Work out the finished part from the listing and answer in its coordinate system (mm). Face numbers are marked on the shaded views. A direction names the side the tool comes from. Give positions to 0.01 mm unless a question says otherwise; leave off trailing zeros. Loops run counter-clockwise (first coordinate to the right, second up) from the corner with the lowest first, then second, coordinate; pieces in that order, holes last. Notation, with made-up numbers: M 61.25,5 L 112.25,5 A12 ccw 112.25,11 Z; hole C 82.5,-7 d2. An arc over 180 degrees is marked long. Use a Markdown table: item, result.
```python
from build123d import *

# Parameters (mm, degrees)
F0_W      = 12
F0_H      = 64
F1_DEPTH  = 2
F2_W      = 2
F2_H      = 32
F3_DEPTH  = 8
F4_W      = 2
F4_H      = 32
F5_DEPTH  = 8
F6_W      = 5
F6_H      = 2
F7_DEPTH  = 5
F8_W      = 5
F8_H      = 1
F9_DEPTH  = 16.501
F10_W     = 2
F10_H     = 32
F11_DEPTH = 24
F12_R     = 1.5
F13_DEPTH = 28.001


with BuildPart() as f1:
    # F0 (on Front) → F1 (new body)
    with BuildSketch(Plane.XZ):
        with Locations((-1.9052418647, 6.8026150874)):
            Rectangle(F0_W, F0_H)
    extrude(amount=F1_DEPTH)

    # F2 (on face) → F3 (join)
    with BuildSketch(Plane.YZ.offset(4.0947581353)):
        with Locations((-1, -9.1973849126)):
            Rectangle(F2_W, F2_H)
    extrude(amount=F3_DEPTH)

    # F4 (on face) → F5 (join)
    with BuildSketch(Plane(origin=(-7.9052418647, 0, 0), x_dir=(0, -1, 0), z_dir=(-1, 0, 0))):
        with Locations((1, -9.1973849126)):
            Rectangle(F4_W, F4_H)
    extrude(amount=F5_DEPTH)

    # F6 (on face) → F7 (join)
    with BuildSketch(Plane.XZ.offset(2)):
        with Locations((-1.9052418647, 38.8026150874)):
            Rectangle(F6_W, F6_H)
    extrude(amount=F7_DEPTH)

    # F8 (on face) → F9 (cut, through all)
    with BuildSketch(Plane(origin=(-4.4052418647, 0, 0), x_dir=(0, -1, 0), z_dir=(-1, 0, 0))):
        with Locations((4.5, 39.3026150874)):
            Rectangle(F8_W, F8_H)
    extrude(amount=-F9_DEPTH, mode=Mode.SUBTRACT)

    # F10 (on face) → F11 (join)
    with BuildSketch(Plane(origin=(0, 0, 0), x_dir=(-1, 0, 0), z_dir=(0, 1, 0))):
        with Locations((-11.0947581353, -9.1973849126)):
            Rectangle(F10_W, F10_H)
        with Locations((14.9052418647, -9.1973849126)):
            Rectangle(F10_W, F10_H)
    extrude(amount=F11_DEPTH)

    # F12 (on face) → F13 (cut, through all)
    with BuildSketch(Plane(origin=(-15.9052418647, 0, 0), x_dir=(0, -1, 0), z_dir=(-1, 0, 0))):
        with Locations((-14, -1.1973849126)):
            Circle(F12_R)
        with Locations((-14, -17.1973849126)):
            Circle(F12_R)
        with BuildLine():
            Line((-23.5, -9.1973849126), (-20.5, -9.1973849126))
            ThreePointArc((-20.5, -9.1973849126), (-22, -7.6973849126), (-23.5, -9.1973849126))
        make_face()
        with BuildLine():
            ThreePointArc((-4.5, -9.1973849126), (-6, -7.6973849126), (-7.5, -9.1973849126))
            Line((-7.5, -9.1973849126), (-4.5, -9.1973849126))
        make_face()
        with BuildLine():
            Line((-4.5, -9.1973849126), (-7.5, -9.1973849126))
            ThreePointArc((-7.5, -9.1973849126), (-6, -10.6973849126), (-4.5, -9.1973849126))
        make_face()
        with BuildLine():
            ThreePointArc((-23.5, -9.1973849126), (-22, -10.6973849126), (-20.5, -9.1973849126))
            Line((-20.5, -9.1973849126), (-23.5, -9.1973849126))
        make_face()
    extrude(amount=-F13_DEPTH, mode=Mode.SUBTRACT)


solid = f1.part
```
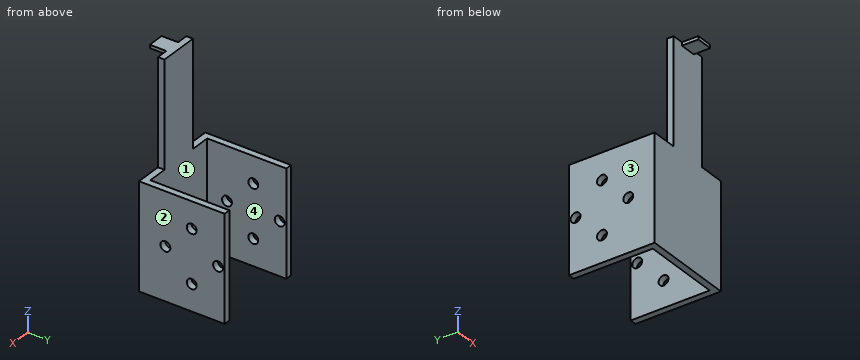
(1) Which of the six approach directions +Z, -Z, +X, -X, +Y, -Y give full straight-line access (tool end or side, diameter ignored) to the marked faces 3 and 4?
Entries:
| item | result |
|---|---|
| face 3 | +Z, -Z, -X, +Y, -Y |
| face 4 | +Z, -Z, +Y |
(2) A cutting plane is placed at D-D (y = 22). Write down the section's boundary in (x, z).
Entries:
| item | result |
|---|---|
| outline | M -15.91,-25.2 L -13.91,-25.2 L -13.91,-10.7 L -15.91,-10.7 Z; M -15.91,-7.7 L -13.91,-7.7 L -13.91,6.8 L -15.91,6.8 Z; M 10.09,-25.2 L 12.09,-25.2 L 12.09,-10.7 L 10.09,-10.7 Z; M 10.09,-7.7 L 12.09,-7.7 L 12.09,6.8 L 10.09,6.8 Z |
(3) Consider probe 1 along Z at (x, y) = (10.95, 14); probe 2 along Z at (x, y) = (11.3, 6); probe 3 along X at (y, z) = (15, 2). Determine where each line is inside the solid, lowest interval first. Write a range as [from, to].
Entries:
| item | result |
|---|---|
| probe 1 | z = [-25.2, -18.7], [-15.7, -2.7], [0.3, 6.8] |
| probe 2 | z = [-25.2, -10.7], [-7.7, 6.8] |
| probe 3 | x = [-15.91, -13.91], [10.09, 12.09] |
(4) A cutting plane is placed at A-A (y = 14). Write down the section's boundary in (x, z), and give its area (3 significant figures).
Entries:
| item | result |
|---|---|
| outline | M -15.91,-25.2 L -13.91,-25.2 L -13.91,-18.7 L -15.91,-18.7 Z; M -15.91,-15.7 L -13.91,-15.7 L -13.91,-2.7 L -15.91,-2.7 Z; M -15.91,0.3 L -13.91,0.3 L -13.91,6.8 L -15.91,6.8 Z; M 10.09,-25.2 L 12.09,-25.2 L 12.09,-18.7 L 10.09,-18.7 Z; M 10.09,-15.7 L 12.09,-15.7 L 12.09,-2.7 L 10.09,-2.7 Z; M 10.09,0.3 L 12.09,0.3 L 12.09,6.8 L 10.09,6.8 Z |
| area | 104 mm² |
(5) The mould has two halves that part along Y. Classify the marked faces 1 and 2: released by +Y, released by -Y, zero draft, split by the parting line, or undercut.
Entries:
| item | result |
|---|---|
| face 1 | released by +Y |
| face 2 | zero draft |
(6) A cutting plane is placed at B-B (y = 1.5). Write down the section's boundary in (x, z).
Entries:
| item | result |
|---|---|
| outline | M -15.91,-25.2 L -13.91,-25.2 L -13.91,6.8 L -15.91,6.8 Z; M 10.09,-25.2 L 12.09,-25.2 L 12.09,6.8 L 10.09,6.8 Z |
(7) A cutting plane is placed at C-C (z = -12). Write down the section's boundary in (x, y).
Entries:
| item | result |
|---|---|
| outline | M -15.91,-2 L 12.09,-2 L 12.09,24 L 10.09,24 L 10.09,0 L -13.91,0 L -13.91,24 L -15.91,24 Z |
(8) Given P1, Ø10, axis at x = 1.5, z = 30.5, coming from the -Y side; P2, Ø12, axis at x = -7, z = -7.5, coming from the +Y side; P3, Ø0.8, axis at y = -4.5, z = 38.5, coming from the +X side; P4, Ø2.5, axis at y = 22, z = -9.2, coming from the +X side, each flat-ended and moving along its own axis, determine where each tip first touches the part or whether it passes through.
Entries:
| item | result |
|---|---|
| P1 | stops at y = -2 |
| P2 | stops at y = 0 |
| P3 | stops at x = 0.59 |
| P4 | passes through |
